Design review of the part shown in the three views and the two pictorial views. Dimensions are in mm from the part's minimum x, y and z. Coordinates: 2 decimals unless noted, no trailing zeros. Write each loop counter-clockwise with the first axis right and the second up, starting at its lowest first coordinate (ties: lowest second). Pieces come first, ordered by that corner, then holes.
Q1. Take a section at C-C, the plane x = 59. Write out the cut boundary in (y, z), plus the area to 3 significant figures.
Q2. Take a section at B-B, the plane y = 16.5. Write out the cut boundary in (x, z), plus the area to 3 significant figures.
Q3. Take a section at A-A, the plane z = 1.3. Write out the cut boundary in (x, y), plus the area to 3 significant figures.
Q4. For pin 1 Ø0.5 at (x, z) = (1, 0.5) entering from -Y; pin 2 Ø1 at (x, z) = (68, 1) entering from -Y; pin 3 Ø1.1 at (x, z) = (0.5, 0.5) entering from +Y, all flat-tipped, find the tip position at first contact; note any pin that passes through.
Q5. For L1, parallel to X at y = 6.5, z = 1.65; L2, parallel to X at y = 16.5, z = 1.1; L3, parallel to Y at x = 67.5, z = 1.9, list the stretches that pass through material, from the lowest coordinate up.
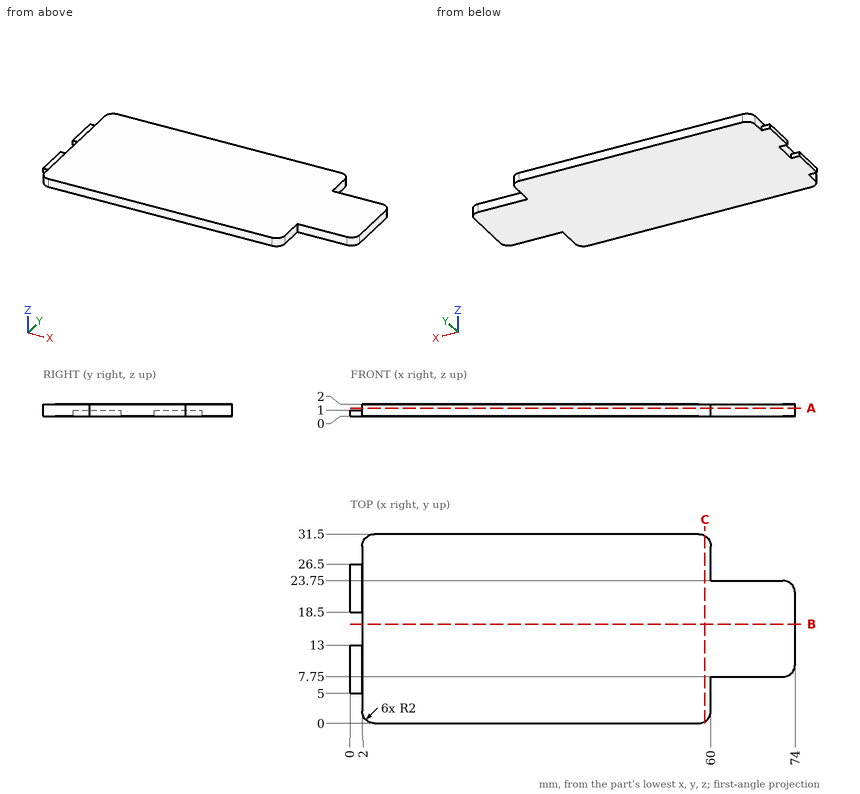
Responses:
1. outline: (0.27, 0) - (31.23, 0) - (31.23, 2) - (0.27, 2) - close
1. area: 61.9 mm2
2. outline: (2, 0) - (74, 0) - (74, 2) - (2, 2) - close
2. area: 144 mm2
3. outline: (2, 2) arc R2 ccw to (4, 0) - (58, 0) arc R2 ccw to (60, 2) - (60, 7.75) - (72, 7.75) arc R2 ccw to (74, 9.75) - (74, 21.75) arc R2 ccw to (72, 23.75) - (60, 23.75) - (60, 29.5) arc R2 ccw to (58, 31.5) - (4, 31.5) arc R2 ccw to (2, 29.5) - close
3. area: 2,050 mm2
4. pin 1: stops at y = 5
4. pin 2: stops at y = 7.75
4. pin 3: stops at y = 26.5
5. L1: x = 2 to 60
5. L2: x = 2 to 74
5. L3: y = 7.75 to 23.75
